```python
from build123d import *

# Parameters (mm, degrees)
SALIENTE_EXTRUIR1_DEPTH      = 3.75
S_LIDO_MOVER_COPIAR2_ANGLE   = 180
S_LIDO_MOVER_COPIAR4_START   = -243.75
S_LIDO_MOVER_COPIAR4_DEPTH   = 7.5
S_LIDO_MOVER_COPIAR4_START_2 = -203.75
S_LIDO_MOVER_COPIAR4_2_DEPTH = 7.5
S_LIDO_MOVER_COPIAR4_START_3 = -123.75
S_LIDO_MOVER_COPIAR4_3_DEPTH = 7.5
S_LIDO_MOVER_COPIAR4_START_4 = -83.75
S_LIDO_MOVER_COPIAR4_4_DEPTH = 7.5
S_LIDO_MOVER_COPIAR5_ANGLE   = 124
S_LIDO_MOVER_COPIAR6_ANGLE   = 120
CROQUIS5_R                   = 6
SALIENTE_EXTRUIR4_DEPTH      = 275
SALIENTE_EXTRUIR5_START      = 146
CROQUIS6_R                   = 6
SALIENTE_EXTRUIR5_DEPTH      = 146
CROQUIS7_R                   = 6
SALIENTE_EXTRUIR6_DEPTH      = 26.25


# Read off the part's stored shape, not the designer's step: Sólido-Mover/Copiar4
with BuildPart() as part:
    # Croquis1 → Saliente-Extruir1 (new, symmetric)
    with BuildSketch(Plane.XY):
        with BuildLine():
            Line((-5.555796523, 15.775), (-10.936607328, 6.053149606))
            ThreePointArc((-10.936607328, 6.053149606), (0, -12.5), (10.936607328, 6.053149606))
            Line((10.936607328, 6.053149606), (5.555796523, 15.775))
            ThreePointArc((5.555796523, 15.775), (0, 19.05), (-5.555796523, 15.775))
        make_face()
    extrude(amount=SALIENTE_EXTRUIR1_DEPTH, both=True)


with BuildPart() as body_2:
    # Sólido-Mover/Copiar1: copy of part
    add(part.part.moved(Location((0, 0, 40))))


with BuildPart() as body_2_1:
    # Sólido-Mover/Copiar2: moved
    add(body_2.part.rotate(Axis((0, 0, 0), (0, 0, 1)), S_LIDO_MOVER_COPIAR2_ANGLE))


with BuildPart() as body_3:
    # Sólido-Mover/Copiar4 outline → Sólido-Mover/Copiar4 (new body)
    with BuildSketch(Plane.XY.offset(S_LIDO_MOVER_COPIAR4_START)):
        with BuildLine():
            ThreePointArc((5.555796523, 15.775), (0, 19.05), (-5.555796523, 15.775))
            Line((-5.555796523, 15.775), (-10.936607328, 6.053149606))
            ThreePointArc((-10.936607328, 6.053149606), (-12.5, 0), (-10.936607328, -6.053149606))
            ThreePointArc((-10.936607328, -6.053149606), (0, -12.5), (10.936607328, -6.053149606))
            ThreePointArc((10.936607328, -6.053149606), (12.5, 0), (10.936607328, 6.053149606))
            Line((10.936607328, 6.053149606), (5.555796523, 15.775))
        make_face()
    extrude(amount=S_LIDO_MOVER_COPIAR4_DEPTH)


with BuildPart() as body_4:
    # S_lido-Mover_Copiar4 2 outline → S_lido-Mover_Copiar4 2 (new body)
    with BuildSketch(Plane.XY.offset(S_LIDO_MOVER_COPIAR4_START_2)):
        with BuildLine():
            Line((-10.936607328, -6.053149606), (-5.555796523, -15.775))
            ThreePointArc((-5.555796523, -15.775), (0, -19.05), (5.555796523, -15.775))
            Line((5.555796523, -15.775), (10.936607328, -6.053149606))
            ThreePointArc((10.936607328, -6.053149606), (0, 12.5), (-10.936607328, -6.053149606))
        make_face()
    extrude(amount=S_LIDO_MOVER_COPIAR4_2_DEPTH)


with BuildPart() as body_5:
    # S_lido-Mover_Copiar4 3 outline → S_lido-Mover_Copiar4 3 (new body)
    with BuildSketch(Plane.XY.offset(S_LIDO_MOVER_COPIAR4_START_3)):
        with BuildLine():
            ThreePointArc((5.555796523, 15.775), (0, 19.05), (-5.555796523, 15.775))
            Line((-5.555796523, 15.775), (-10.936607328, 6.053149606))
            ThreePointArc((-10.936607328, 6.053149606), (-12.5, 0), (-10.936607328, -6.053149606))
            ThreePointArc((-10.936607328, -6.053149606), (0, -12.5), (10.936607328, -6.053149606))
            ThreePointArc((10.936607328, -6.053149606), (12.5, 0), (10.936607328, 6.053149606))
            Line((10.936607328, 6.053149606), (5.555796523, 15.775))
        make_face()
    extrude(amount=S_LIDO_MOVER_COPIAR4_3_DEPTH)


with BuildPart() as body_6:
    # S_lido-Mover_Copiar4 4 outline → S_lido-Mover_Copiar4 4 (new body)
    with BuildSketch(Plane.XY.offset(S_LIDO_MOVER_COPIAR4_START_4)):
        with BuildLine():
            Line((-10.936607328, -6.053149606), (-5.555796523, -15.775))
            ThreePointArc((-5.555796523, -15.775), (0, -19.05), (5.555796523, -15.775))
            Line((5.555796523, -15.775), (10.936607328, -6.053149606))
            ThreePointArc((10.936607328, -6.053149606), (0, 12.5), (-10.936607328, -6.053149606))
        make_face()
    extrude(amount=S_LIDO_MOVER_COPIAR4_4_DEPTH)


with BuildPart() as body_6_1:
    # Sólido-Mover/Copiar5: moved
    add(body_6.part.rotate(Axis((0, 0, 0), (0, 0, 1)), S_LIDO_MOVER_COPIAR5_ANGLE))


with BuildPart() as body_5_1:
    # Sólido-Mover/Copiar5: moved
    add(body_5.part.rotate(Axis((0, 0, 0), (0, 0, 1)), S_LIDO_MOVER_COPIAR5_ANGLE))


with BuildPart() as body_3_1:
    # Sólido-Mover/Copiar6: moved
    add(body_3.part.rotate(Axis((0, 0, 0), (0, 0, -1)), S_LIDO_MOVER_COPIAR6_ANGLE))


with BuildPart() as body_4_1:
    # Sólido-Mover/Copiar6: moved
    add(body_4.part.rotate(Axis((0, 0, 0), (0, 0, -1)), S_LIDO_MOVER_COPIAR6_ANGLE))


with BuildPart() as part_1:
    add(part.part)

    add(body_2_1.part)  # Saliente-Extruir4 merges body 2

    add(body_3_1.part)  # Saliente-Extruir4 merges body 3

    add(body_4_1.part)  # Saliente-Extruir4 merges body 4

    add(body_5_1.part)  # Saliente-Extruir4 merges body 5

    add(body_6_1.part)  # Saliente-Extruir4 merges body 6
    # Croquis5 → Saliente-Extruir4 (add)
    with BuildSketch(Plane.XY.offset(-236.25)):
        Circle(CROQUIS5_R)
    extrude(amount=SALIENTE_EXTRUIR4_DEPTH)

    # Croquis6 → Saliente-Extruir5 (add)
    with BuildSketch(Plane(origin=(0, 0, -243.75), x_dir=(-1, 0, 0), z_dir=(0, 0, -1)).offset(SALIENTE_EXTRUIR5_START)):
        with Locations(Location((0, 0, 0), (0, 0, 180))):
            Circle(CROQUIS6_R)
    extrude(amount=-SALIENTE_EXTRUIR5_DEPTH)

    # Croquis7 → Saliente-Extruir6 (add)
    with BuildSketch(Plane.XY.offset(43.75)):
        Circle(CROQUIS7_R)
    extrude(amount=SALIENTE_EXTRUIR6_DEPTH)


solid = part_1.part
```
Read the model definition and answer for the solid it produces. Units are mm, in the model's axes. A direction names the side the tool comes from. Round coordinates to 2 decimals unless told otherwise and drop trailing zeros. Write each loop counter-clockwise with the first axis right and the second up, starting at its lowest first coordinate (ties: lowest second). Pieces come first, ordered by that corner, then holes. Notation, with made-up numbers: (63.25, -5.75) - (78.25, -5.75) arc R19 ccw to (78.25, 17.25) - close; hole circle Ø10 at (73.5, 60). An arc over 180 degrees is marked (long way). One line per item, written item: value.
Q1. Each of these flat-tipped pins is pushed along its axis until it touches: P1, Ø1, axis at y = -2.5, z = -328.5, coming from the -X side; P2, Ø1.5, axis at x = 3.5, z = -47.5, coming from the +Y side; P3, Ø12, axis at x = 2.5, y = 14, coming from the -Z side. Where does it stop, or does it pass through?
The answers:
P1: stops at x = -5.66
P2: stops at y = 5.33
P3: stops at z = -243.75
Q2. Find section A-A (z = -278). Determine the outline of the cut face in (x, y), and give its area (3 significant figures).
The answers:
outline: circle Ø12 at (0, 0)
area: 113 mm2
Q3. For a pull along Z with two mould halves and no side action, classify faces 1 (the cylindrical face through (-6, 0, 20)), 2 (the flat face through (-13.624, 0.803, -120.052)), 3 (the flat face through (0, 0, 70)) as pulls with the +Z half, pulls with the -Z half, needs draft (parallel to the pull), parting line crosses it, or undercut.
The answers:
face 1: undercut
face 2: needs draft
face 3: pulls with the +Z half
Q4. Which of the six approach directions +Z, -Z, +X, -X, +Y, -Y give full straight-line access (tool end or side, diameter ignored) to faces 4 (the flat face through (-4.514, -12.946, -120.052)), 5 (the flat face through (8.28, 10.85, 0.05)), 6 (the flat face through (6, 4, -76.25)), 7 (the flat face through (-8.28, -10.85, 40.05)), 8 (the flat face through (0, -7, 43.75))?
The answers:
face 4: -Z, +X, -Y
face 5: +Z, +X, +Y
face 6: none
face 7: +Z, -X, -Y
face 8: +Z
Q5. Straight lines are drawn through the part: line 1 (Z direction, x = -7.5, y = 4); line 2 (Z direction, x = -8, y = 12); line 3 (X direction, y = 0.5, z = -182.5). For each, find the intervals that lie inside material, in ascending order. Write a range as from..to.
The answers:
line 1: z = -243.75..-236.25, -203.75..-196.25, -123.75..-116.25, -83.75..-76.25, -3.75..3.75, 36.25..43.75
line 2: z = -203.75..-196.25
line 3: x = -5.98..5.98
